Build history of the part. All positions in model axes, mm. A direction names the side the tool comes from. Coordinates: 2 decimals unless noted, no trailing zeros. Write each loop counter-clockwise with the first axis right and the second up, starting at its lowest first coordinate (ties: lowest second). Pieces come first, ordered by that corner, then holes.
Autodesk Inventor part; units mm, degrees
ref_plane "Work Plane2" through (3.35, 0, 0) normal (0, 0, -1) x (1, 0, 0)
ref_plane "YZ Plane" through (0, 0, 0) normal (1, 0, 0) x (0, 1, 0)
ref_plane "XZ Plane" through (0, 0, 0) normal (0, 1, 0) x (-1, 0, 0)
sketch "Sketch1" plane through (0, 0, 0) normal (0, 0, 1) x (1, 0, 0)
  line L0 (3.2, 0) -> (14, 0)
  line L1 (14, 0) -> (14, 2.5)
  line L2 (14, 2.5) -> (4.3, 2.5)
  line L3 (4.3, 2.5) -> (3.8092, 2.2546)
  line L4 (3.8092, 2.2546) -> (2.7, 2.2546)
  line L5 (0, 4.65) -> (0, 2.6)
  line L6 (0, 2.6) -> (2.4732, 1.3669)
  line L7 (2.4732, 1.3669) -> (3.2, 0)
  line L8 (-2.8, 0) -> (16.8, 0)
  line L9 (0, -0.93) -> (0, 5.58)
  line L10 (0, 4.65) -> (0.3046, 4.65)
  line L11 (0.3046, 4.65) -> (2.7, 2.2546)
  line L12 (4.3, 2.5) -> (2.4546, 2.5) construction
  dimension "d1" = 9.7
  dimension "d2" = 5
  dimension "d3" = 4.5092
  dimension "d4" = 5.2
  dimension "d5" = 26.5
  dimension "d6" = 62
  dimension "d7" = 3.2
  dimension "d8" = 0.4908
  dimension "d12" = 9.3
  dimension "d13" = 45
  dimension "d15" = 14
  dimension "d24" = 2.7
revolve "Body" add sketch "Sketch1" angle 360 about axis through (3.2, 0, 0) along (1, 0, 0) contours L7 L6 L5 L10 L11 L4 L3 L2 L1 L0
sketch "Sketch2" plane through (0, 0, 0) normal (-1, 0, 0) x (0, 0, 1)
  line L0 (0, 2.6) -> (0, 0) construction
  line L1 (0, 0) -> (2.6, 0) construction
  arc A0 (0.78, 0) -> (0, 0.78) centre (0, 0) ccw construction
  arc A1 (0.91, 0) -> (0, 0.91) centre (0, 0) ccw construction
  arc A2 (2.579, 0.33) -> (0.33, 2.579) centre (0, 0) ccw
  line L2 (0, 0) -> (1.8385, 1.8385) construction
  line L3 (0.33, 2.579) -> (0.4413, 0.7958)
  line L4 (2.579, 0.33) -> (0.7958, 0.4413)
  arc A3 (0.33, 2.579) -> (0, 2.6) centre (0, 0) ccw
  arc A4 (2.6, 0) -> (2.579, 0.33) centre (0, 0) ccw
  line L5 (0, -6.51) -> (0, 6.51)
  line L6 (-6.51, 0) -> (6.51, 0)
  arc A5 (0.33, -2.579) -> (2.579, -0.33) centre (0, 0) ccw
  line L7 (0.33, -2.579) -> (0.4413, -0.7958)
  line L8 (2.579, -0.33) -> (0.7958, -0.4413)
  arc A6 (0, -2.6) -> (0.33, -2.579) centre (0, 0) ccw
  arc A7 (2.579, -0.33) -> (2.6, 0) centre (0, 0) ccw
  arc A8 (-0.33, 2.579) -> (-2.579, 0.33) centre (0, 0) ccw
  line L9 (-0.33, 2.579) -> (-0.4413, 0.7958)
  line L10 (-2.579, 0.33) -> (-0.7958, 0.4413)
  arc A9 (0, 2.6) -> (-0.33, 2.579) centre (0, 0) ccw
  arc A10 (-2.579, 0.33) -> (-2.6, 0) centre (0, 0) ccw
  arc A11 (-0.33, -2.579) -> (0, -2.6) centre (0, 0) ccw
  arc A12 (-2.579, -0.33) -> (-0.33, -2.579) centre (0, 0) ccw
  arc A13 (-2.6, 0) -> (-2.579, -0.33) centre (0, 0) ccw
  line L11 (-2.579, -0.33) -> (-0.7958, -0.4413)
  line L12 (-0.33, -2.579) -> (-0.4413, -0.7958)
  arc A14 (0.4413, 0.7958) -> (0.7958, 0.4413) centre (0.8194, 0.8194) ccw
  arc A15 (0.7958, -0.4413) -> (0.4413, -0.7958) centre (0.8194, -0.8194) ccw
  arc A16 (-0.7958, 0.4413) -> (-0.4413, 0.7958) centre (-0.8194, 0.8194) ccw
  arc A17 (-0.4413, -0.7958) -> (-0.7958, -0.4413) centre (-0.8194, -0.8194) ccw
  point P0 (1.8385, -1.8385)
  point P1 (-1.8385, 1.8385)
  point P2 (-1.8385, -1.8385)
  dimension "d17" = 1.56
  dimension "d18" = 1.82
  dimension "d19" = 5.2
  dimension "d20" = 45
  dimension "d21" = 0.33
extrude "Slot" add sketch "Sketch2" against normal up to next draft 5 contours L4 A14 L3 A2 | A5 L7 A15 L8 | L9 A16 L10 A8 | A12 L11 A17 L12
fillet "Fillet1" radius 0.132 4 edges at (0, 2.6, 0) (0, 0, -2.6) (0, -2.6, 0) (0, 0, 2.6)
thread "Thread"
chamfer "Chamfer1" distance 0.4908 distance2 0.2454 1 edges at (14, -2.5, 0) measured on face at (14, 0.1959, -0.44)
ref_plane "Work Plane2" through (3.35, 0, 0) normal (0, 0, -1) x (1, 0, 0)
equation "\"d1\" = GEL"
equation "\"d2\" = GD"
equation "\"d3\" = BDM"
equation "\"d4\" = SDM"
equation "\"d7\" = INTI"
equation "\"d8\" = GAL"
equation "\"d12\" = KOD"
equation "\"d13\" = 0.5 * SEWI"
equation "\"d15\" = NLG"
equation "\"d24\" = KOH"
equation "\"d17\" = 0.3 * SDM"
equation "\"d18\" = 0.35 * SDM"
equation "\"d19\" = SDM"
equation "\"d21\" = 0.5 * SBR"
equation "\"d23\" = 0.2 * SBR"
equation "\"d10\" = GEL"
equation "\"d25\" = -0.5 * SPD + 0.5 * GD"
equation "\"d26\" = 0.5 * GAL"
equation "\"NLG\" = 14"
equation "\"GEL\" = 9.7"
equation "\"GAL\" = 0.61345 * PTC"
equation "\"SPD\" = NND - 1.2269 * PTC"
equation "\"KOD\" = 9.3"
equation "\"KOH\" = 2.7"
equation "\"SBR\" = 0.66"
equation "\"INTI\" = 3.2"
equation "\"SDM\" = 5.2"
equation "\"GD\" = NND"
equation "\"BDM\" = NND - GAL"
equation "\"SEWI\" = 90deg"
equation "\"d9\" = SDM"
equation "\"GUL\" = 0.61345 * PTC"
equation "\"TOA\" = 30deg"
equation "\"EPV\" = 5.2"
equation "\"THREADDIA\" = 5"
equation "\"PTC\" = 0.8"
equation "\"NND\" = 5"
equation "\"GD1\" = THREADDIA - 1.2269 * PTC"
properties part number "ISO 7046-1 - M5 x 14 - 4.8 - H" material "Steel"
1. 3-axis set-ups, long thin cutter, end or side, ignore diameter. For faces 1 (the face through (3.25, 2.15, -0.68)), 2 (the face through (0.154, 2.5, 3.921)), 3 (the face through (1.26, 0, 1.97)): which of +Z, -Z, +X, -X, +Y, -Y reach the whole face in a straight line?
Computed values:
face 1: none
face 2: +X, -X
face 3: -X
2. Saw through at B-B on x = 12. List the corners of the cut face in (y, z).
Computed values:
outline: circle Ø5 at (0, 0)
3. Saw through at A-A on x = 2.25. List the corners of the cut face in (y, z), plus the area to 3 significant figures.
Computed values:
outline: circle Ø5.41 at (0, 0); hole (-1.46, -0.2) - (-0.78, -0.24) arc R0.58 cw to (-0.24, -0.78) - (-0.2, -1.46) arc R1.48 ccw to (0.2, -1.46) - (0.24, -0.78) arc R0.58 cw to (0.78, -0.24) - (1.46, -0.2) arc R1.48 ccw to (1.46, 0.2) - (0.78, 0.24) arc R0.58 cw to (0.24, 0.78) - (0.2, 1.46) arc R1.48 ccw to (-0.2, 1.46) - (-0.24, 0.78) arc R0.58 cw to (-0.78, 0.24) - (-1.46, 0.2) arc R1.48 ccw to start
area: 20.2 mm2
4. Probe line 1 along Y through (x, z) = (2, 0); line 2 along X through (y, z) = (-0.75, -2.25); line 3 along Z through (x, y) = (11.5, 0). List the from-to ranges inside material, lowest first.
Computed values:
line 1: y = -2.95 to -1.6, 1.6 to 2.95
line 2: x = 0 to 2.58, 4.04 to 13.82
line 3: z = -2.5 to 2.5
5. Flat gauge pins, fed straight in: pin 1 (3 mm diameter, centred on x = 5, z = -1, fed in from -Y); pin 2 (5 mm diameter, centred on x = 2.5, z = 2.5, fed in from +Y); pin 3 (3 mm diameter, centred on x = 10, y = -3.5, fed in from +Z). Where does each tip first touch, or does it go through?
Computed values:
pin 1: stops at y = -2.5
pin 2: stops at y = 4.46
pin 3: stops at z = 1.5
6. Mould opens along Z. For faces 4 (the face through (2.55, -0.313, -2.384)), 5 (the face through (1.058, -1.321, -0.316)), 6 (the face through (0, 1, -1)), 7 (the face through (1.058, 0.316, -1.321)) say: +Z half, -Z half, draft (parallel to the pull), parting line (faces both ways), or undercut.
Computed values:
face 4: parting line
face 5: undercut
face 6: draft
face 7: undercut
